Could you check a few things on this model? Use its own coordinates, in mm. Face numbers are marked on the shaded views. A direction names the side the tool comes from. Give positions to 0.01 mm unless a question says otherwise; leave off trailing zeros. Loops run counter-clockwise (first coordinate to the right, second up) from the corner with the lowest first, then second, coordinate; pieces in that order, holes last. Notation, with made-up numbers: (78, 1.25) -> (133, 1.25) arc R21 cw to (133, 29.25) -> close; hole circle Ø5 at (69, 7.25). An arc over 180 degrees is marked (long way). Write item = value, one per line. Start each with the question number.
1) I need wall thicknesses on probe 1 along Y at (x, z) = (-9, -9.5); probe 2 along X at (y, z) = (41, -8); probe 3 along Y at (x, z) = (30.5, -16). Which ranges of each line are inside material? Lowest first, please. Write a range as from..to.
2) If we mould it in two halves opening along Y, with no side actions, what happens to the marked faces 4, 5 and 6? For each: +Y half, -Y half, draft (parallel to the pull), parting line (faces both ways), or undercut.
3) I want a section at A-A (z = -9.5). List the corners of the cut face in (x, y) for me.
4) I want a section at D-D (z = 9.5). List the corners of the cut face in (x, y) for me.
5) I want a section at B-B (x = -8.5). List the corners of the cut face in (y, z) for me.
6) I'm going to push flat-ended pins straight in: pin 1 Ø12 at (y, z) = (38, -0.5) entering from +X; pin 2 Ø12 at (x, z) = (2.5, 10.5) entering from -Y. Where does each tip first touch, or does it pass through?
7) I want a section at C-C (y = 29). List the corners of the cut face in (x, z) for me.
8) On a 3-axis mill with a long thin cutter (end or side, diameter ignored), from which of +Z, -Z, +X, -X, +Y, -Y can I reach the whole of each face in a straight line? I mean the marked faces 1, 2 and 3. Say none if no direction works.
from build123d import *

# Parameters (mm, degrees)
SKETCH1_W               = 70
SKETCH1_H               = 40
BOSS_EXTRUDE1_DEPTH     = 60
SKETCH2_W               = 30
SKETCH2_H               = 10
CUT_EXTRUDE1_DEPTH      = 81.156097709
SKETCH3_W               = 10
SKETCH3_H               = 20
CUT_EXTRUDE2_DEPTH      = 81.156097709
CUT_EXTRUDE3_DEPTH      = 81.156097709
CUT_EXTRUDE3_DEPTH_BACK = 20


with BuildPart() as part:
    # Sketch1 → Boss-Extrude1 (new body)
    with BuildSketch(Plane(origin=(0, 0, 0), x_dir=(1, 0, 0), z_dir=(0, 1, 0))):
        Rectangle(SKETCH1_W, SKETCH1_H)
    extrude(amount=BOSS_EXTRUDE1_DEPTH)

    # Sketch2 → Cut-Extrude1 (cut, through all)
    with BuildSketch(Plane.XY.offset(20)):
        with Locations((0, 5)):
            Rectangle(SKETCH2_W, SKETCH2_H)
    extrude(amount=-CUT_EXTRUDE1_DEPTH, mode=Mode.SUBTRACT)

    # Sketch3 → Cut-Extrude2 (cut, through all)
    with BuildSketch(Plane.XY.offset(20)):
        with Locations((30, 40)):
            Rectangle(SKETCH3_W, SKETCH3_H)
    extrude(amount=-CUT_EXTRUDE2_DEPTH, mode=Mode.SUBTRACT)

    # Sketch4 → Cut-Extrude3 (cut, two sides: drawn at the far end of the back side and taken through both)
    with BuildSketch(Plane.XY.offset(20).offset(-CUT_EXTRUDE3_DEPTH_BACK)):
        Polygon((-156.088610322, -101.088610322), (-35, 20), (5, 60), (126.088610322, 181.088610322), (-116.088610322, 423.265830965), (-398.265830965, 141.088610322), align=None)
    extrude(amount=CUT_EXTRUDE3_DEPTH + CUT_EXTRUDE3_DEPTH_BACK, mode=Mode.SUBTRACT)


solid = part.part
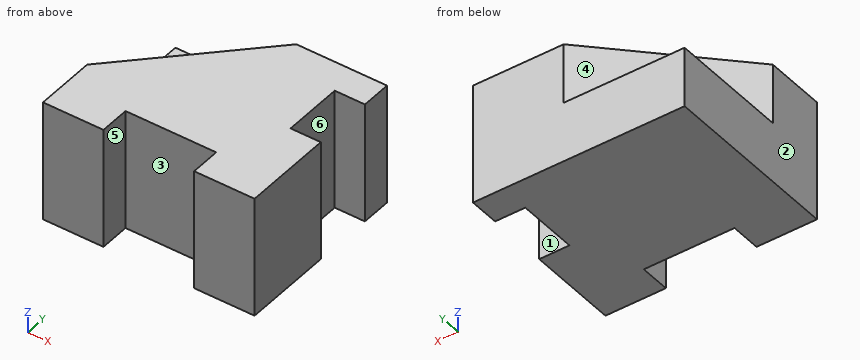
Answer list:
q1.probe_1 = 10..60
q1.probe_2 = -35..25
q1.probe_3 = 0..30, 50..60
q2.face_4 = +Y half
q2.face_5 = draft
q2.face_6 = undercut
q3.outline = (-35, 0) -> (-15, 0) -> (-15, 10) -> (15, 10) -> (15, 0) -> (35, 0) -> (35, 30) -> (25, 30) -> (25, 50) -> (35, 50) -> (35, 60) -> (-35, 60) -> close
q4.outline = (-35, 0) -> (-15, 0) -> (-15, 10) -> (15, 10) -> (15, 0) -> (35, 0) -> (35, 30) -> (25, 30) -> (25, 50) -> (35, 50) -> (35, 60) -> (5, 60) -> (-35, 20) -> close
q5.outline = (10, -20) -> (60, -20) -> (60, 0) -> (46.5, 0) -> (46.5, 20) -> (10, 20) -> close
q6.pin_1 = 25
q6.pin_2 = 10
q7.outline = (-35, -20) -> (35, -20) -> (35, 20) -> (-26, 20) -> (-26, 0) -> (-35, 0) -> close
q8.face_1 = +Z, -Z, +X
q8.face_2 = +Z, -Z, -X, +Y, -Y
q8.face_3 = +Z, -Z, -Y
